from build123d import *
from build123d.topology import SkipClean

# Parameters (mm, degrees)
EXTRUDE_1_DEPTH           = 20
SKETCH_3_R                = 5.5
CUT_EXTRUDE_2_DEPTH       = 10
SKETCH_9_R                = 6.25
CUT_EXTRUDE_6_DEPTH       = 1
SKETCH_11_W               = 20
SKETCH_11_H               = 5
EXTRUDE_4_DEPTH           = 10
CUT_EXTRUDE_8_REACH       = 78.472
SKETCH_12_R               = 1.5
SKETCH_13_R               = 3
CUT_EXTRUDE_9_DEPTH       = 2.5
SKETCH_14_R               = 10
SKETCH_14_R_2             = 5.5
EXTRUDE_5_DEPTH           = 6
CUT_EXTRUDE_START         = -1
SKETCH_6_R                = 6.25
CUT_EXTRUDE_10_DEPTH      = 1
SKETCH_15_W               = 20
SKETCH_15_H               = 5
EXTRUDE_6_DEPTH           = 5
SKETCH_16_W               = 17
SKETCH_16_H               = 3
EXTRUDE_7_DEPTH           = 15
CUT_EXTRUDE_11_DEPTH      = 70.961190435
CUT_EXTRUDE_11_DEPTH_BACK = 70.961190435
EXTRUDE_START             = -5
SKETCH_3D_3_R             = 1.5
EXTRUDE_8_DEPTH           = 5
CUT_EXTRUDE_12_DEPTH      = 2.5
FILLET_1_R                = 2
CUT_EXTRUDE_14_DEPTH      = 76.06644022
SKETCH_21_W               = 6.587713241
SKETCH_21_H               = 4.5
EXTRUDE_9_DEPTH           = 15
SKETCH_23_W               = 25
SKETCH_23_H               = 20
CUT_EXTRUDE_16_DEPTH      = 5
CUT_EXTRUDE_17_DEPTH      = 10


with BuildPart() as part:
    # 草图1 → 凸台-拉伸1 (new body)
    with BuildSketch(Plane.XY):
        Polygon((-63.866818046, 22.947717095), (-23.866818046, 22.947717095), (-23.866818046, -19.052282905), (-33.866818046, -19.052282905), (-33.866818046, 14.947717095), (-63.866818046, 14.947717095), align=None)
    extrude(amount=EXTRUDE_1_DEPTH)

    # 草图3 → 切除-拉伸2 (cut)
    with BuildSketch(Plane(origin=(0, 22.947717095, 0), x_dir=(-1, 0, 0), z_dir=(0, 1, 0))):
        with Locations((50.866818046, 10)):
            Circle(SKETCH_3_R)
    extrude(amount=-CUT_EXTRUDE_2_DEPTH, mode=Mode.SUBTRACT)

    # 草图9 → 切除-拉伸6 (cut)
    with BuildSketch(Plane(origin=(0, 22.947717095, 0), x_dir=(1, 0, 0), z_dir=(0, 1, 0))):
        with Locations(Location((-50.866818046, -10, 0), (0, 0, 180))):
            Circle(SKETCH_9_R)
    extrude(amount=-CUT_EXTRUDE_6_DEPTH, mode=Mode.SUBTRACT)

    # 草图11 → 凸台-拉伸4 (add)
    with BuildSketch(Plane(origin=(-23.866818046, 0, 0), x_dir=(0, 0, -1), z_dir=(1, 0, 0))):
        with Locations((-10, -16.552282905)):
            Rectangle(SKETCH_11_W, SKETCH_11_H)
    extrude(amount=EXTRUDE_4_DEPTH)

    # 草图12 → 切除-拉伸8 (cut, up to next)
    with BuildSketch(Plane(origin=(0, -14.052282905, 0), x_dir=(-1, 0, 0), z_dir=(0, 1, 0)), mode=Mode.PRIVATE) as cut_extrude_8_sk1:
        with Locations((18.866818046, 5)):
            Circle(SKETCH_12_R)
    cut_extrude_8_tool1 = extrude(cut_extrude_8_sk1.sketch, amount=-CUT_EXTRUDE_8_REACH, mode=Mode.PRIVATE) & part.part
    # 草图12 → 切除-拉伸8 (cut, up to next)
    with BuildSketch(Plane(origin=(0, -14.052282905, 0), x_dir=(-1, 0, 0), z_dir=(0, 1, 0)), mode=Mode.PRIVATE) as cut_extrude_8_sk2:
        with Locations((18.866818046, 15)):
            Circle(SKETCH_12_R)
    cut_extrude_8_tool2 = extrude(cut_extrude_8_sk2.sketch, amount=-CUT_EXTRUDE_8_REACH, mode=Mode.PRIVATE) & part.part
    add(cut_extrude_8_tool1.solids().sort_by_distance((-18.866818, -14.052283, 5))[0], mode=Mode.SUBTRACT)
    add(cut_extrude_8_tool2.solids().sort_by_distance((-18.866818, -14.052283, 15))[0], mode=Mode.SUBTRACT)

    # 草图13 → 切除-拉伸9 (cut)
    with BuildSketch(Plane.XZ.offset(19.052282905)):
        with Locations(Location((-18.866818046, 15, 0), (0, 0, 270))):
            Circle(SKETCH_13_R)
        with Locations(Location((-18.866818046, 5, 0), (0, 0, 270))):
            Circle(SKETCH_13_R)
    extrude(amount=-CUT_EXTRUDE_9_DEPTH, mode=Mode.SUBTRACT)

    # 草图14 → 凸台-拉伸5 (add)
    with SkipClean():  # the faces are left unmerged after this step: merging them gives an invalid solid
        with BuildSketch(Plane.XZ.offset(-14.947717095)):
            with Locations(Location((-50.866818046, 10, 0), (0, 0, 270))):
                Circle(SKETCH_14_R)
            with Locations(Location((-50.866818046, 10, 0), (0, 0, 180))):
                Circle(SKETCH_14_R_2, mode=Mode.SUBTRACT)
        extrude(amount=EXTRUDE_5_DEPTH)

    # 草图6 → 切除-拉伸10 (cut)
    with BuildSketch(Plane.XZ.offset(-8.947717095).offset(CUT_EXTRUDE_START)):
        with Locations(Location((-50.866818046, 10, 0), (0, 0, 180))):
            Circle(SKETCH_6_R)
    extrude(amount=CUT_EXTRUDE_10_DEPTH, mode=Mode.SUBTRACT)

    # 草图15 → 凸台-拉伸6 (add)
    with BuildSketch(Plane(origin=(-13.866818046, 0, 0), x_dir=(0, 0, -1), z_dir=(1, 0, 0))):
        with Locations((-10, -16.552282905)):
            Rectangle(SKETCH_15_W, SKETCH_15_H)
    extrude(amount=EXTRUDE_6_DEPTH)

    # 草图16 → 凸台-拉伸7 (add)
    with BuildSketch(Plane.XZ.offset(-14.947717095)):
        with Locations((-42.366818046, 18.5)):
            Rectangle(SKETCH_16_W, SKETCH_16_H)
        with Locations((-42.366818046, 1.5)):
            Rectangle(SKETCH_16_W, SKETCH_16_H)
    extrude(amount=EXTRUDE_7_DEPTH)

    # 草图17 → 切除-拉伸11 (cut, two sides: drawn at the far end of the back side and taken through both)
    with BuildSketch(Plane(origin=(0, 0, 17), x_dir=(-1, 0, 0), z_dir=(0, 0, -1)).offset(-CUT_EXTRUDE_11_DEPTH_BACK)):
        Polygon((50.866818046, 8.947717095), (43.725389617, 8.947717095), (33.866818046, -0.052282905), (50.866818046, -0.052282905), align=None)
    extrude(amount=CUT_EXTRUDE_11_DEPTH + CUT_EXTRUDE_11_DEPTH_BACK, mode=Mode.SUBTRACT)

    # Sketch 3D_3 → 凸台-拉伸8 (add)
    with BuildSketch(Plane(origin=(-23.866818046, -6.052282905, 20), x_dir=(0.447213595499958, 0, -0.894427190999916), z_dir=(0, -1, 0)).offset(EXTRUDE_START)):
        Polygon((0, 0), (4.472135955, 8.94427191), (22.360679775, 0), (17.88854382, -8.94427191), align=None)
        with Locations(Location((6.708203932, 2.236067977, 0), (0, 0, 243.434948823))):
            Circle(SKETCH_3D_3_R, mode=Mode.SUBTRACT)
        with Locations(Location((15.652475842, -2.236067977, 0), (0, 0, 243.434948823))):
            Circle(SKETCH_3D_3_R, mode=Mode.SUBTRACT)
    extrude(amount=EXTRUDE_8_DEPTH)

    # 草图18 → 切除-拉伸12 (cut)
    with BuildSketch(Plane(origin=(0, -1.052282905, 0), x_dir=(-1, 0, 0), z_dir=(0, 1, 0))):
        Polygon((15.691391565, 15), (17.279104805, 12.25), (20.454531286, 12.25), (22.042244526, 15), (20.454531286, 17.75), (17.279104805, 17.75), align=None)
        Polygon((15.691391565, 5), (17.279104805, 2.25), (20.454531286, 2.25), (22.042244526, 5), (20.454531286, 7.75), (17.279104805, 7.75), align=None)
    extrude(amount=-CUT_EXTRUDE_12_DEPTH, mode=Mode.SUBTRACT)

    # 圆角1
    # the kernel refuses this fillet: 2 mm, written as the material it adds along each edge
    with BuildSketch(Plane(origin=(-23.866818046, -1.052282905, 0), x_dir=(0, 1, 0), z_dir=(0, 0, 1))) as fillet_1_piece_1_section:
        with BuildLine():
            CenterArc((FILLET_1_R, -FILLET_1_R), FILLET_1_R, 90, 90)
            Line((0, -FILLET_1_R), (0, 0))
            Line((0, 0), (FILLET_1_R, 0))
        make_face()
    fillet_1_piece_1 = extrude(amount=20, mode=Mode.PRIVATE)
    fillet_1_piece_1 = split(fillet_1_piece_1, bisect_by=Plane(origin=(-20.802583542, -0.671658343, 2.852844192), z_dir=(-0.8660254037844387, 0, -0.5000000000000001)), keep=Keep.TOP, mode=Mode.PRIVATE)
    fillet_1_piece_1 = split(fillet_1_piece_1, bisect_by=Plane(origin=(-23.907001975, -0.671658343, 1.770145354), z_dir=(0.8660254037844387, 0, -0.5000000000000003)), keep=Keep.TOP, mode=Mode.PRIVATE)
    add(fillet_1_piece_1)
    with BuildSketch(Plane(origin=(-23.866818046, -1.052282905, 0), x_dir=(0, 1, 0), z_dir=(0, 0, 1))) as fillet_1_piece_2_section:
        with BuildLine():
            CenterArc((FILLET_1_R, -FILLET_1_R), FILLET_1_R, 90, 90)
            Line((0, -FILLET_1_R), (0, 0))
            Line((0, 0), (FILLET_1_R, 0))
        make_face()
    fillet_1_piece_2 = extrude(amount=20, mode=Mode.PRIVATE)
    fillet_1_piece_2 = split(fillet_1_piece_2, bisect_by=Plane(origin=(-22.4188867, -0.519681884, 5.652363381), z_dir=(-0.8660254037844387, 0, -0.5000000000000001)), keep=Keep.TOP, mode=Mode.PRIVATE)
    fillet_1_piece_2 = split(fillet_1_piece_2, bisect_by=Plane(origin=(-22.4188867, -0.519681884, 4.347636619), z_dir=(-0.8660254037844387, 0, 0.5000000000000003)), keep=Keep.TOP, mode=Mode.PRIVATE)
    add(fillet_1_piece_2)
    with BuildSketch(Plane(origin=(-23.866818046, -1.052282905, 0), x_dir=(0, 1, 0), z_dir=(0, 0, 1))) as fillet_1_piece_3_section:
        with BuildLine():
            CenterArc((FILLET_1_R, -FILLET_1_R), FILLET_1_R, 90, 90)
            Line((0, -FILLET_1_R), (0, 0))
            Line((0, 0), (FILLET_1_R, 0))
        make_face()
    fillet_1_piece_3 = extrude(amount=20, mode=Mode.PRIVATE)
    fillet_1_piece_3 = split(fillet_1_piece_3, bisect_by=Plane(origin=(-24.519856268, -0.671658343, 9.291349419), z_dir=(0.8660254037844387, 0, 0.5000000000000001)), keep=Keep.TOP, mode=Mode.PRIVATE)
    fillet_1_piece_3 = split(fillet_1_piece_3, bisect_by=Plane(origin=(-20.189729249, -0.671658343, 8.208650581), z_dir=(-0.8660254037844387, 0, 0.5000000000000003)), keep=Keep.TOP, mode=Mode.PRIVATE)
    fillet_1_piece_3 = split(fillet_1_piece_3, bisect_by=Plane(origin=(-20.189729249, -0.671658343, 11.791349419), z_dir=(-0.8660254037844387, 0, -0.5)), keep=Keep.TOP, mode=Mode.PRIVATE)
    fillet_1_piece_3 = split(fillet_1_piece_3, bisect_by=Plane(origin=(-24.519856268, -0.671658343, 10.708650581), z_dir=(0.8660254037844384, 0, -0.5000000000000004)), keep=Keep.TOP, mode=Mode.PRIVATE)
    add(fillet_1_piece_3)
    with BuildSketch(Plane(origin=(-23.866818046, -1.052282905, 0), x_dir=(0, 1, 0), z_dir=(0, 0, 1))) as fillet_1_piece_4_section:
        with BuildLine():
            CenterArc((FILLET_1_R, -FILLET_1_R), FILLET_1_R, 90, 90)
            Line((0, -FILLET_1_R), (0, 0))
            Line((0, 0), (FILLET_1_R, 0))
        make_face()
    fillet_1_piece_4 = extrude(amount=20, mode=Mode.PRIVATE)
    fillet_1_piece_4 = split(fillet_1_piece_4, bisect_by=Plane(origin=(-22.4188867, -0.519681884, 15.652363381), z_dir=(-0.8660254037844387, 0, -0.5)), keep=Keep.TOP, mode=Mode.PRIVATE)
    fillet_1_piece_4 = split(fillet_1_piece_4, bisect_by=Plane(origin=(-22.4188867, -0.519681884, 14.347636619), z_dir=(-0.8660254037844384, 0, 0.5000000000000004)), keep=Keep.TOP, mode=Mode.PRIVATE)
    add(fillet_1_piece_4)
    with BuildSketch(Plane(origin=(-23.866818046, -1.052282905, 0), x_dir=(0, 1, 0), z_dir=(0, 0, 1))) as fillet_1_piece_5_section:
        with BuildLine():
            CenterArc((FILLET_1_R, -FILLET_1_R), FILLET_1_R, 90, 90)
            Line((0, -FILLET_1_R), (0, 0))
            Line((0, 0), (FILLET_1_R, 0))
        make_face()
    fillet_1_piece_5 = extrude(amount=20, mode=Mode.PRIVATE)
    fillet_1_piece_5 = split(fillet_1_piece_5, bisect_by=Plane(origin=(-23.907001975, -0.671658343, 18.229854646), z_dir=(0.8660254037844387, 0, 0.5)), keep=Keep.TOP, mode=Mode.PRIVATE)
    fillet_1_piece_5 = split(fillet_1_piece_5, bisect_by=Plane(origin=(-20.802583542, -0.671658343, 17.147155808), z_dir=(-0.8660254037844384, 0, 0.5000000000000004)), keep=Keep.TOP, mode=Mode.PRIVATE)
    add(fillet_1_piece_5)

    # 草图20 → 切除-拉伸14 (cut, through all)
    with SkipClean():  # the faces are left unmerged after this step: merging them gives an invalid solid
        with BuildSketch(Plane.XZ.offset(-14.947717095)):
            with BuildLine():
                Line((-63.866818046, 20), (-50.866818046, 20))
                ThreePointArc((-50.866818046, 20), (-60.866818046, 10), (-50.866818046, 0))
                Line((-50.866818046, 0), (-63.866818046, 0))
                Line((-63.866818046, 0), (-63.866818046, 20))
            make_face()
        extrude(amount=-CUT_EXTRUDE_14_DEPTH, mode=Mode.SUBTRACT)
    add(part.part.scale(1), mode=Mode.REPLACE)  # the faces are merged on a copy

    # 草图21 → 凸台-拉伸9 (add)
    with BuildSketch(Plane(origin=(0, -1.052282905, 0), x_dir=(1, 0, 0), z_dir=(0, 1, 0))):
        with Locations((-20.572961426, -10)):
            Rectangle(SKETCH_21_W, SKETCH_21_H)
    extrude(amount=EXTRUDE_9_DEPTH)

    # 草图23 → 切除-拉伸16 (cut)
    with BuildSketch(Plane.XZ.offset(19.052282905)):
        with Locations((-21.366818046, 10)):
            Rectangle(SKETCH_23_W, SKETCH_23_H)
    extrude(amount=-CUT_EXTRUDE_16_DEPTH, mode=Mode.SUBTRACT)

    # 草图24 → 切除-拉伸17 (cut)
    with BuildSketch(Plane.XY.offset(12.25)):
        Polygon((-23.866818046, 13.947717095), (-17.279104805, -1.052282905), (-17.279104805, 13.947717095), align=None)
    extrude(amount=-CUT_EXTRUDE_17_DEPTH, mode=Mode.SUBTRACT)


solid = part.part
Source: CAD feature listing. Evaluate the final solid. Frame: model axes, mm. A direction names the side the tool comes from. Give positions to 0.01 mm unless a question says otherwise; leave off trailing zeros. Order: outer loops, then holes, each group sorted by start corner. A loop starts at its lowest first (then second) coordinate and runs counter-clockwise, first axis right, second up. Notation, with made-up numbers: (85, 76) -> (137, 76) arc R26 cw to (137, 106) -> close; hole circle Ø1 at (1, 0). An arc over 180 degrees is marked (long way). Use a Markdown table: item, result.
1) Section query D-D, the plane x = -42. Return the cut outline in (y, z), then the cut area to 3 significant figures.
Answer list:
| item | result |
|---|---|
| outline | (7.37, 0) -> (22.95, 0) -> (22.95, 20) -> (7.37, 20) -> (7.37, 17) -> (14.95, 17) -> (14.95, 14.62) -> (8.95, 14.62) -> (8.95, 5.38) -> (14.95, 5.38) -> (14.95, 3) -> (7.37, 3) -> close |
| area | 261 mm² |
2) Ray query, line 1 along X through (y, z) = (14, 5); line 2 along X through (y, z) = (9.7, 10); line 3 along Y through (x, z) = (-34, 9.75). Return the intervals inside material, ascending. Write a range as [from, to].
Answer list:
| item | result |
|---|---|
| line 1 | [-59.53, -53.16], [-48.58, -42.21], [-33.87, -23.87] |
| line 2 | [-60.87, -57.12], [-44.62, -40.87], [-33.87, -22] |
| line 3 | [14.95, 22.95] |
3) Section query A-A, the plane z = 10. Return the cut outline in (x, y).
Answer list:
| item | result |
|---|---|
| outline | (-60.87, 8.95) -> (-57.12, 8.95) -> (-57.12, 9.95) -> (-56.37, 9.95) -> (-56.37, 21.95) -> (-57.12, 21.95) -> (-57.12, 22.95) -> (-60.87, 22.95) -> close; (-45.37, 9.95) -> (-44.62, 9.95) -> (-44.62, 8.95) -> (-40.87, 8.95) -> (-40.87, 14.95) -> (-33.87, 14.95) -> (-33.87, -14.05) -> (-23.87, -14.05) -> (-23.87, -6.05) -> (-13.87, -6.05) -> (-13.87, -1.05) -> (-17.28, -1.05) -> (-23.87, 13.95) -> (-23.87, 22.95) -> (-44.62, 22.95) -> (-44.62, 21.95) -> (-45.37, 21.95) -> close |
4) Mould query, pull axis X, two halves, no side actions, for faces 5 (the cylindrical face through (-20.298, -4.785, 4.549)), 6 (the flat face through (-23.867, -10, 10)), 7 (the cylindrical face through (-60.864, 15.85, 10.22)). Classes: +X half, -X half, draft (parallel to the pull), parting line (faces both ways), or undercut.
Answer list:
| item | result |
|---|---|
| face 5 | undercut |
| face 6 | +X half |
| face 7 | -X half |
5) Reachability of faces 1 (the flat face through (-23.867, 15, 10)), 2 (the flat face through (-16.5, -2.3, 16.4)), 3 (the flat face through (-33.867, 0, 10)), 4 (the flat face through (-21.4, -1.052, 13)) from +Z, -Z, +X, -X, +Y, -Y: full face, straight path, thin tool, end or side. Return the list, or none.
Answer list:
| item | result |
|---|---|
| face 1 | +X, +Y |
| face 2 | +Y |
| face 3 | -Y |
| face 4 | +Z, +X, +Y |
6) Section query B-B, the plane y = 4. Return the cut outline in (x, z), then the cut area to 3 significant figures.
Answer list:
| item | result |
|---|---|
| outline | (-38.31, 0) -> (-23.87, 0) -> (-23.87, 7.75) -> (-19.5, 7.75) -> (-19.5, 12.25) -> (-23.87, 12.25) -> (-23.87, 20) -> (-38.31, 20) -> (-38.31, 17) -> (-33.87, 17) -> (-33.87, 3) -> (-38.31, 3) -> close |
| area | 246 mm² |
7) Section query C-C, the plane x = -21. Return the cut outline in (y, z), then the cut area to 3 significant figures.
Answer list:
| item | result |
|---|---|
| outline | (-6.05, 0) -> (-1.05, 0) -> (-1.05, 3.19) -> (-3.55, 3.19) -> (-3.55, 6.81) -> (-1.05, 6.81) -> (-1.05, 7.75) -> (7.42, 7.75) -> (7.42, 12.25) -> (-1.05, 12.25) -> (-1.05, 13.19) -> (-3.55, 13.19) -> (-3.55, 16.81) -> (-1.05, 16.81) -> (-1.05, 20) -> (-6.05, 20) -> close |
| area | 120 mm² |
8) Contact query for flat-ended pins moving along their axis: P1, Ø5, axis at x = -18.5, z = 10, coming from the -Y side; P2, Ø3, axis at y = -9, z = 12.5, coming from the -X side; P3, Ø10, axis at x = -50.87, z = 10, coming from the +Y side; P4, Ø8, axis at x = -39.5, z = 10, coming from the -Y side. Output: stop coordinate, or through.
Answer list:
| item | result |
|---|---|
| P1 | y = -6.05 |
| P2 | x = -33.87 |
| P3 | through |
| P4 | y = 8.95 |
